```python
from build123d import *

# Parameters (mm, degrees)
BOSS_EXTRUDE1_DEPTH = 6.35
SKETCH2_R           = 1
CUT_EXTRUDE1_DEPTH  = 12.7
CUT_EXTRUDE2_DEPTH  = 3.55
CUT_EXTRUDE3_START  = -6.35
CUT_EXTRUDE3_DEPTH  = 3


with BuildPart() as part:
    # Sketch1 → Boss-Extrude1 (new, symmetric)
    with BuildSketch(Plane.XY):
        with BuildLine():
            Line((0, 5), (40, 5))
            ThreePointArc((40, 5), (45, 0), (40, -5))
            Line((40, -5), (0, -5))
            ThreePointArc((0, -5), (-5, 0), (0, 5))
        make_face()
    extrude(amount=BOSS_EXTRUDE1_DEPTH, both=True)

    # Sketch2 → Cut-Extrude1 (cut)
    with BuildSketch(Plane.XY.offset(6.35)):
        with Locations((40, 0)):
            Circle(SKETCH2_R)
        Circle(SKETCH2_R)
    extrude(amount=-CUT_EXTRUDE1_DEPTH, mode=Mode.SUBTRACT)

    # Sketch3 → Cut-Extrude2 (cut)
    with BuildSketch(Plane.XY.offset(6.35)):
        with BuildLine():
            Line((35, 5), (35, -5))
            Line((35, -5), (40, -5))
            ThreePointArc((40, -5), (45, 0), (40, 5))
            Line((40, 5), (35, 5))
        make_face()
    cut_extrude2 = extrude(amount=-CUT_EXTRUDE2_DEPTH, mode=Mode.SUBTRACT)

    # Mirror1: Cut-Extrude2 across plane
    add(cut_extrude2.mirror(Plane.XY), mode=Mode.SUBTRACT)

    # Sketch4 → Cut-Extrude3 (cut, symmetric)
    with BuildSketch(Plane.XY.offset(6.35).offset(CUT_EXTRUDE3_START)):
        with BuildLine():
            Line((5, 5), (5, -5))
            Line((5, -5), (0, -5))
            ThreePointArc((0, -5), (-5, 0), (0, 5))
            Line((0, 5), (5, 5))
        make_face()
    extrude(amount=CUT_EXTRUDE3_DEPTH, both=True, mode=Mode.SUBTRACT)


solid = part.part
```
For this review, take the finished solid that the model builds, in its own axes (mm). A direction names the side the tool comes from. Round coordinates to 2 decimals unless told otherwise and drop trailing zeros. Write each loop counter-clockwise with the first axis right and the second up, starting at its lowest first coordinate (ties: lowest second). Pieces come first, ordered by that corner, then holes. Notation, with made-up numbers: (-2, 82.5) - (11, 82.5) arc R26 ccw to (11, 109.5) - close; hole circle Ø4 at (82, 57.25). An arc over 180 degrees is marked (long way). Answer as CSV lines item,"result". Start each with the question number.
(1) Mouldability with a two-part tool opening along Y and no side actions: class faces 1 (the cylindrical face through (0, -1, 5)), 2 (the cylindrical face through (41, 0, 0)), 3 (the cylindrical face through (-5, 0, 5)), 4 (the flat face through (35, 0, 5)) as +Y half, -Y half, draft (parallel to the pull), parting line (faces both ways), or undercut.
(2) Add section B-B, the plane z = -5.25. State the section outline as (x, y) points.
(3) For pin 1 (3 mm diameter, centred on y = 0, z = -0.5, fed in from -X); pin 2 (3 mm diameter, centred on x = 41.5, y = -1.5, fed in from -Z); pin 3 (1.5 mm diameter, centred on y = 2.5, z = -2.5, fed in from +X); pin 4 (1.8 mm diameter, centred on x = 40, y = 0, fed in from -Z), all flat-tipped, find the tip position at first contact; note any pin that passes through.
(4) Add section D-D, the plane y = -2. State the section outline as (x, z) points.
(5) For line 1 (Z direction, x = 2.5, y = -3); line 2 (Y direction, x = 0, z = 5.5); line 3 (Z direction, x = 38, y = 1.25), list the stretches that pass through material, from the lowest coordinate up.
(6) Add section A-A, the plane y = 0. State the section outline as (x, z) points, plus the area to 3 significant figures.
(7) Machinability: for faces 5 (the flat face through (38.8, 0.1, 2.8)), 6 (the cylindrical face through (-5, 0, -5)), 7 (the flat face through (20, -5, 0)), 8 (the flat face through (38.8, 0.1, -2.8)), 9 (the flat face through (1.2, 0.1, -3)), which of the approach directions +Z, -Z, +X, -X, +Y, -Y give a long, thin tool a straight path to every point of the face, cutting with its end or side? Answer none if there is none.
(8) Add section C-C, the plane y = 2.25. State the section outline as (x, z) points.
From the geometry:
1,face 1,"undercut"
1,face 2,"undercut"
1,face 3,"parting line"
1,face 4,"draft"
2,outline,"(0, -5) - (35, -5) - (35, 5) - (0, 5) arc R5 ccw to start; hole circle Ø2 at (0, 0)"
3,pin 1,"stops at x = 5"
3,pin 2,"stops at z = -2.8"
3,pin 3,"stops at x = 44.68"
3,pin 4,"passes through"
4,outline,"(-4.58, -6.35) - (35, -6.35) - (35, -2.8) - (44.58, -2.8) - (44.58, 2.8) - (35, 2.8) - (35, 6.35) - (-4.58, 6.35) - (-4.58, 3) - (5, 3) - (5, -3) - (-4.58, -3) - close"
5,line 1,"z = -6.35 to -3, 3 to 6.35"
5,line 2,"y = -5 to -1, 1 to 5"
5,line 3,"z = -2.8 to 2.8"
6,outline,"(-5, -6.35) - (-1, -6.35) - (-1, -3) - (-5, -3) - close; (-5, 3) - (-1, 3) - (-1, 6.35) - (-5, 6.35) - close; (1, -6.35) - (35, -6.35) - (35, -2.8) - (39, -2.8) - (39, 2.8) - (35, 2.8) - (35, 6.35) - (1, 6.35) - (1, 3) - (5, 3) - (5, -3) - (1, -3) - close; (41, -2.8) - (45, -2.8) - (45, 2.8) - (41, 2.8) - close"
6,area,"479 mm²"
7,face 5,"+Z, +X, +Y, -Y"
7,face 6,"+Z, -Z, -X"
7,face 7,"+Z, -Z, +X, -X, -Y"
7,face 8,"-Z, +X, +Y, -Y"
7,face 9,"-X, +Y, -Y"
8,outline,"(-4.47, -6.35) - (35, -6.35) - (35, -2.8) - (44.47, -2.8) - (44.47, 2.8) - (35, 2.8) - (35, 6.35) - (-4.47, 6.35) - (-4.47, 3) - (5, 3) - (5, -3) - (-4.47, -3) - close"
